Read the model definition and answer for the solid it produces. Units are mm, in the model's axes. A direction names the side the tool comes from. Round coordinates to 2 decimals unless told otherwise and drop trailing zeros. Order: outer loops, then holes, each group sorted by start corner. A loop starts at its lowest first (then second) coordinate and runs counter-clockwise, first axis right, second up. Notation, with made-up numbers: (17, 1) - (32, 1) arc R26 ccw to (32, 24) - close; hole circle Ø1 at (32, 76). An arc over 180 degrees is marked (long way). Put each result on its own line as item: value. Start each with the question number.
Q1. Section A-A on y = -5.25 is taken. Give the vertices of the cut face in (x, z).
Q2. Section C-C on z = 0 is taken. Give the vertices of the cut face in (x, y), then the cut area to 3 significant figures.
Q3. Section B-B on x = -12 is taken. Give the vertices of the cut face in (y, z), then the cut area to 4 significant figures.
Q4. Section D-D on x = 0 is taken. Give the vertices of the cut face in (y, z), then the cut area to 3 significant figures.
Q5. Find the intervals of material crossed by line 1 along Z through (x, y) = (31.5, 2.5); line 2 along Z through (x, y) = (-21.5, -6.5); line 3 along X through (y, z) = (-9, -21), in increasing order. Write a range as from..to.
Q6. Each of these flat-tipped pins is pushed along its axis until it touches: pin 1 Ø2 at (x, z) = (-18, -39.5) entering from -Y; pin 2 Ø8 at (x, y) = (-22.5, 7.5) entering from -Z; pin 3 Ø1.5 at (y, z) = (8.5, 30.5) entering from -X; pin 4 Ø3.5 at (x, y) = (15, 9) entering from +Z. Where does it stop, or does it pass through?
Q7. For a pull along X with two mould halves and no side action, classify faces 1 (the face through (33.46, -9.01, 48.37)), 2 (the face through (33.64, 7.97, -48.57)), 3 (the face through (-35, -2, -50)) as pulls with the +X half, pulls with the -X half, needs draft (parallel to the pull), parting line crosses it, or undercut.
Q8. Which of the six approach directions +Z, -Z, +X, -X, +Y, -Y give full straight-line access (tool end or side, diameter ignored) to faces 4 (the face through (35, -2, -50)), 5 (the face through (33.37, -9.01, -48.46)), 6 (the face through (17, 9, 42.5))?
Autodesk Inventor part; units mm, degrees
ref_plane "YZ Plane" through (0, 0, 0) normal (1, 0, 0) x (0, 1, 0)
ref_plane "XZ Plane" through (0, 0, 0) normal (0, 1, 0) x (-1, 0, 0)
ref_plane "XY Plane" through (0, 0, 0) normal (0, 0, 1) x (1, 0, 0)
sketch "Sketch5" plane through (0, 0, 0) normal (1, 0, 0) x (0, 1, 0)
  line L0 (10, 52.5) -> (-10, 52.5)
  line L1 (-10, 52.5) -> (-10, -52.5)
  line L2 (-10, -52.5) -> (10, -52.5)
  line L3 (10, -52.5) -> (10, 52.5)
  point P0 (0, 0)
  point P1 (10, 0)
  point P2 (0, -52.5)
  dimension "d6" = 20
  dimension "d30" = 105
extrude "Extrusion2" add sketch "Sketch5" along normal mid plane 75
shell "Shell1" thickness 3 removed faces 1 at (-12.5, -10, 17.5)
chamfer "Chamfer4" distance 5 angle 45 8 edges at (37.5, 0, 52.5) (34.5, -1.5, 49.5) (34.5, -1.5, -49.5) (37.5, 0, -52.5) (-37.5, 0, -52.5) (-34.5, -1.5, -49.5) (-37.5, 0, 52.5) (-34.5, -1.5, 49.5)
sketch "Sketch7" plane through (-37.5, -10, -52.5) normal (0, -1, 0) x (1, 0, 0)
  line L0 (3, 8) -> (3, 97)
  line L1 (8, 102) -> (67, 102)
  line L2 (72, 97) -> (72, 8)
  line L3 (67, 3) -> (8, 3)
  line L4 (5, 0) -> (70, 0)
  line L5 (75, 100) -> (75, 5)
  line L6 (5, 105) -> (70, 105)
  line L7 (0, 5) -> (0, 100)
  line L8 (8, 102) -> (3, 97)
  line L9 (72, 97) -> (67, 102)
  line L10 (67, 3) -> (72, 8)
  line L11 (3, 8) -> (8, 3)
  line L12 (0, 100) -> (5, 105)
  line L13 (5, 0) -> (0, 5)
  line L14 (75, 5) -> (70, 0)
  line L15 (70, 105) -> (75, 100)
  line L16 (67.8284, 104) -> (7.1716, 104)
  line L17 (7.1716, 104) -> (1, 97.8284)
  line L18 (1, 97.8284) -> (1, 7.1716)
  line L19 (1, 7.1716) -> (7.1716, 1)
  line L20 (7.1716, 1) -> (67.8284, 1)
  line L21 (67.8284, 1) -> (74, 7.1716)
  line L22 (74, 7.1716) -> (74, 97.8284)
  line L23 (74, 97.8284) -> (67.8284, 104)
  dimension "d61" = 2
extrude "Extrusion4" cut sketch "Sketch7" against normal blind 2 contours L23 L22 L21 L20 L19 L18 L17 L16
sketch "Sketch8" plane through (-37.5, 10, 52.5) normal (0, 1, 0) x (1, 0, 0)
  line L0 (32, 10) -> (10, 10)
  line L1 (10, 10) -> (10, 28.5)
  line L2 (10, 28.5) -> (32, 28.5)
  line L3 (32, 28.5) -> (32, 10)
  line L4 (32, 10) -> (10, 28.5) construction
  line L5 (10, 10) -> (32, 28.5) construction
  line L6 (0, 0) -> (0, 105)
  line L7 (75, 0) -> (0, 0)
  point P0 (37.5, 52.5)
  point P1 (21, 19.25)
  dimension "d35" = 22
  dimension "d36" = 18.5
  dimension "d49" = 10
  dimension "d54" = 10
extrude "Extrusion5" cut sketch "Sketch8" against normal blind 3
mirror "Mirror4" about plane through (0, 0, 0) normal (1, 0, 0) of "Extrusion5"
sketch "Sketch9" plane through (37.5, 0, 0) normal (1, 0, 0) x (0, 0, -1)
  circle A0 centre (0, 0) radius 3.5
  circle A1 centre (0, 0) radius 8.5 construction
  line L0 (-8.5, 0) -> (8.5, 0) construction
  line L1 (8.5, 0) -> (8.5, -13) construction
  line L2 (8.5, -13) -> (-8.5, -13) construction
  line L3 (-8.5, -13) -> (-8.5, 0) construction
  dimension "d43" = 17
  dimension "d41" = 7
  dimension "d45" = 13
  dimension "d46" = 0
extrude "Extrusion6" cut sketch "Sketch9" against normal blind 3
pattern_linear "Rectangular Pattern1" count 2 spacing 25 along (0, 0, -1) of "Extrusion6"
chamfer "Chamfer5" distance 4 angle 45 8 edges at (37.5, 10, 0) (35, 10, 50) (0, 10, 52.5) (-35, 10, 50) (-37.5, 10, 0) (-35, 10, -50) (0, 10, -52.5) (35, 10, -50)
sketch "Sketch10" plane through (32.5, -10, -52.5) normal (0, 0, -1) x (-1, 0, 0)
  line L0 (0, 16) -> (65, 16)
  line L1 (0, 0) -> (0, 16)
  line L2 (65, 0) -> (0, 0)
  line L3 (65, 16) -> (65, 0)
  point P0 (32.5, 10)
  point P1 (32.5, 4.75)
  dimension "d65" = 4.75
hole "Hole1" at (0, -5.25, -52.5) direction (0, 0, 1) diameter 3 depth 5
mirror "Mirror5" about plane through (0, 0, 0) normal (0, 0, 1) of "Hole1"
properties part number "Casing-v2-top"
Findings:
1. outline: (-37.5, -47.5) - (-32.5, -52.5) - (-1.5, -52.5) - (-1.5, -49.5) - (-29.5, -49.5) - (-34.5, -44.5) - (-34.5, 44.5) - (-29.5, 49.5) - (-1.5, 49.5) - (-1.5, 52.5) - (-32.5, 52.5) - (-37.5, 47.5) - close; (1.5, -52.5) - (32.5, -52.5) - (37.5, -47.5) - (37.5, 47.5) - (32.5, 52.5) - (1.5, 52.5) - (1.5, 49.5) - (29.5, 49.5) - (34.5, 44.5) - (34.5, -44.5) - (29.5, -49.5) - (1.5, -49.5) - close
2. outline: (-37.5, -10) - (-36.5, -10) - (-36.5, -8) - (-34.5, -8) - (-34.5, 7) - (34.5, 7) - (34.5, 3.5) - (37.5, 3.5) - (37.5, 6) - (33.5, 10) - (-33.5, 10) - (-37.5, 6) - close; (34.5, -8) - (36.5, -8) - (36.5, -10) - (37.5, -10) - (37.5, -3.5) - (34.5, -3.5) - close
2. area: 282 mm2
3. outline: (-10, -52.5) - (6, -52.5) - (10, -48.5) - (10, 24) - (7, 24) - (7, -49.5) - (-8, -49.5) - (-8, -51.5) - (-10, -51.5) - close; (-10, 51.5) - (-8, 51.5) - (-8, 49.5) - (7, 49.5) - (7, 42.5) - (10, 42.5) - (10, 48.5) - (6, 52.5) - (-10, 52.5) - close
3. area: 337.5 mm2
4. outline: (-10, -52.5) - (-6.75, -52.5) - (-6.75, -49.5) - (-8, -49.5) - (-8, -51.5) - (-10, -51.5) - close; (-10, 51.5) - (-8, 51.5) - (-8, 49.5) - (-6.75, 49.5) - (-6.75, 52.5) - (-10, 52.5) - close; (-3.75, -52.5) - (6, -52.5) - (10, -48.5) - (10, 48.5) - (6, 52.5) - (-3.75, 52.5) - (-3.75, 49.5) - (7, 49.5) - (7, -49.5) - (-3.75, -49.5) - close
4. area: 375 mm2
5. line 1: -52.5..-47.5, 47.5..52.5
5. line 2: -52.5..-49.5, 49.5..52.5
5. line 3: -37.5..-36.5, 36.5..37.5
6. pin 1: y = 7
6. pin 2: z = -52.5
6. pin 3: x = -35.75
6. pin 4: z = 51.25
7. face 1: undercut
7. face 2: pulls with the +X half
7. face 3: pulls with the -X half
8. face 4: -Z, +X, +Y, -Y
8. face 5: -Y
8. face 6: +Y, -Y
